The model under review builds one solid part; all positions refer to its coordinate system, in mm. Give positions to 0.01 mm unless a question says otherwise; leave off trailing zeros. Order: outer loops, then holes, each group sorted by start corner. A loop starts at its lowest first (then second) coordinate and runs counter-clockwise, first axis right, second up.
```python
from build123d import *

# Parameters (mm, degrees)
SKETCH_1_R      = 2.013000515
SKETCH_1_R_2    = 1.5
EXTRUDE_2_DEPTH = 6


with BuildPart() as part:
    # 草图1 → 凸台-拉伸2 (new body)
    # profile 1 of 2: a face of its own
    with BuildSketch(Plane(origin=(0, 0, 0), x_dir=(1, 0, 0), z_dir=(0, 1, 0))):
        with BuildLine():
            ThreePointArc((158.5, 0), (160, 1.5), (161.5, 0))
            Line((161.5, 0), (172.5, 0))
            ThreePointArc((172.5, 0), (0, 172.5), (-172.5, 0))
            Line((-172.5, 0), (-161.5, 0))
            ThreePointArc((-161.5, 0), (-160, 1.5), (-158.5, 0))
            Line((-158.5, 0), (-114, 0))
            Line((-114, 0), (-114, 45))
            Line((-114, 45), (-74, 45))
            Line((-74, 45), (-74, 22.705919103))
            Line((-74, 22.705919103), (74, 22.705919103))
            Line((74, 22.705919103), (74, 45))
            Line((74, 45), (114, 45))
            Line((114, 45), (114, 0))
            Line((114, 0), (158.5, 0))
        make_face()
        with Locations(Location((-12, 127.620399327, 0), (0, 0, 270))):
            Circle(SKETCH_1_R, mode=Mode.SUBTRACT)
        with Locations(Location((-80, 138.564064606, 0), (0, 0, 270))):
            Circle(SKETCH_1_R_2, mode=Mode.SUBTRACT)
        with Locations(Location((-12, 157.620399327, 0), (0, 0, 270))):
            Circle(SKETCH_1_R, mode=Mode.SUBTRACT)
        with Locations(Location((12, 127.620399327, 0), (0, 0, 270))):
            Circle(SKETCH_1_R, mode=Mode.SUBTRACT)
        with Locations(Location((12, 157.620399327, 0), (0, 0, 270))):
            Circle(SKETCH_1_R, mode=Mode.SUBTRACT)
        with Locations(Location((80, 138.564064606, 0), (0, 0, 270))):
            Circle(SKETCH_1_R_2, mode=Mode.SUBTRACT)
    # profile 2 of 2: a face of its own
    with BuildSketch(Plane(origin=(0, 0, 0), x_dir=(1, 0, 0), z_dir=(0, 1, 0))):
        with BuildLine():
            Line((172.5, 0), (161.5, 0))
            ThreePointArc((161.5, 0), (160, -1.5), (158.5, 0))
            Line((158.5, 0), (114, 0))
            Line((114, 0), (114, -45))
            Line((114, -45), (74, -45))
            Line((74, -45), (74, -22.705919103))
            Line((74, -22.705919103), (-74, -22.705919103))
            Line((-74, -22.705919103), (-74, -45))
            Line((-74, -45), (-114, -45))
            Line((-114, -45), (-114, 0))
            Line((-114, 0), (-158.5, 0))
            ThreePointArc((-158.5, 0), (-160, -1.5), (-161.5, 0))
            Line((-161.5, 0), (-172.5, 0))
            ThreePointArc((-172.5, 0), (0, -172.5), (172.5, 0))
        make_face()
        with Locations(Location((-80, -138.564064606, 0), (0, 0, 270))):
            Circle(SKETCH_1_R_2, mode=Mode.SUBTRACT)
        with Locations(Location((80, -138.564064606, 0), (0, 0, 270))):
            Circle(SKETCH_1_R_2, mode=Mode.SUBTRACT)
    extrude(amount=-EXTRUDE_2_DEPTH)


solid = part.part
```
1. To check wall thickness, follow line 1 (Z direction, x = 80, y = -4.1); line 2 (X direction, y = -5.4, z = 40); line 3 (X direction, y = -4.65, z = 43). State the ranges of each line that lie inside material, in increasing order.
2. Take a section at D-D (z = -69). Write out the cut boundary in (x, y).
3. Take a section at C-C (x = 36.5). Write out the cut boundary in (y, z).
4. Take a section at A-A (x = 0). Write out the cut boundary in (y, z), and give its area (3 significant figures).
5. Take a section at B-B (y = -1.1). Count the separate pieces of the cut face and the enclosed holes in it, and give its area (3 significant figures).
6. Insertion check: pin 1 (6.5 mm diameter, centred on x = -12, z = -157.62, fed in from -Y); pin 2 (3 mm diameter, centred on x = -35.5, y = -3.5, fed in from +Z); pin 3 (1.5 mm diameter, centred on y = -0.5, z = 42.5, fed in from +X); pin 4 (1.5 mm diameter, centred on x = 109, y = -2, fed in from +Z). Each pin has a flat end and moves straight along its axis. Give the tip position at first contact, or say it passes through.
Answer:
1. line 1: z = -152.83 to -140.06, -137.06 to -45, 45 to 137.06, 140.06 to 152.83
1. line 2: x = -167.8 to -114, -74 to 74, 114 to 167.8
1. line 3: x = -167.05 to -114, -74 to 74, 114 to 167.05
2. outline: (-158.1, -6) - (158.1, -6) - (158.1, 0) - (-158.1, 0) - close
3. outline: (-6, -168.59) - (0, -168.59) - (0, -22.71) - (-6, -22.71) - close; (-6, 22.71) - (0, 22.71) - (0, 168.59) - (-6, 168.59) - close
4. outline: (-6, -172.5) - (0, -172.5) - (0, -22.71) - (-6, -22.71) - close; (-6, 22.71) - (0, 22.71) - (0, 172.5) - (-6, 172.5) - close
4. area: 1,800 mm2
5. separate pieces: 1
5. enclosed holes: 11
5. area: 79,500 mm2
6. pin 1: stops at y = -6
6. pin 2: stops at z = 169.12
6. pin 3: stops at x = 167.37
6. pin 4: stops at z = 134.31
